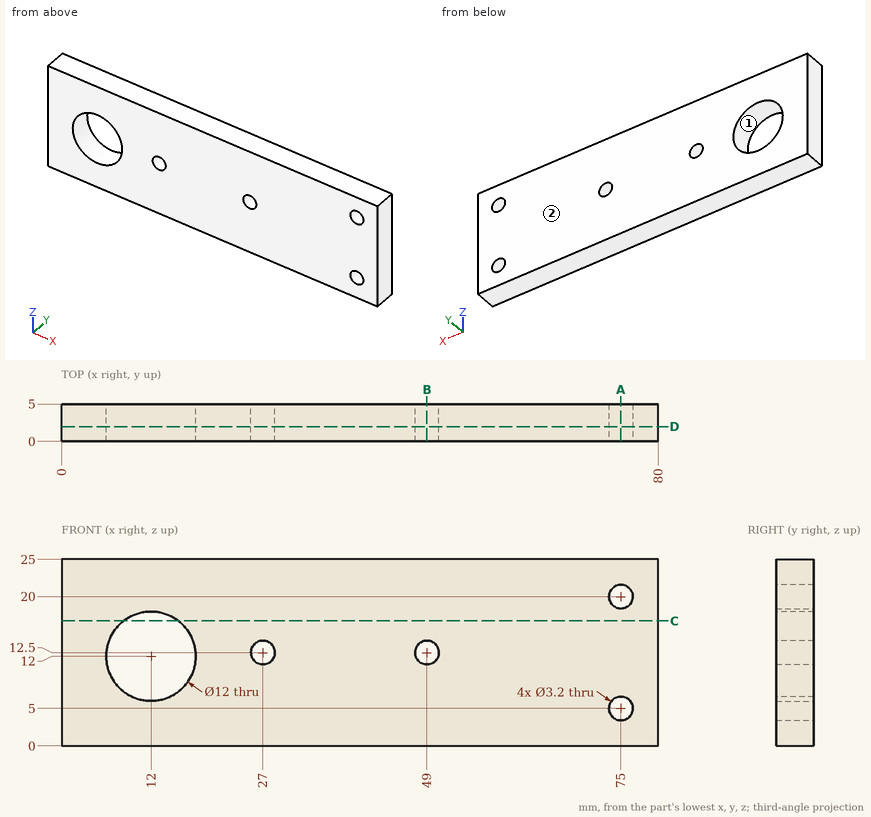
Drawing for the job (mm, zero at the part's lowest x, y, z). Coordinates: 2 decimals unless noted, no trailing zeros. Write each loop counter-clockwise with the first axis right and the second up, starting at its lowest first coordinate (ties: lowest second). Pieces come first, ordered by that corner, then holes. Notation, with made-up numbers: (-32, 69.25) - (-14, 69.25) arc R33 ccw to (-14, 98.25) - close; hole circle Ø8 at (6.25, 52.5). An arc over 180 degrees is marked (long way). Write each question's results on one line, items separated by ' | '. Start each with the question number.
1) Cut at C-C (z = 16.75). Write the cut outline in (x, y), then the cut area to 3 significant figures.
2) Cut at B-B (x = 49). Write the cut outline in (y, z).
3) Flat gauge pin, fed straight in: P1, Ø3, axis at x = 27, z = 12.5, coming from the +Y side. Where does the tip first touch, or does it go through?
4) Probe line 1 along Z through (x, y) = (75, 3.6); line 2 along X through (y, z) = (2.55, 20); line 3 along Z through (x, y) = (12, 3). List the from-to ranges inside material, lowest first. Write a range as from..to.
5) Cut at D-D (y = 1.95). Write the cut outline in (x, z).
6) Mould opens along X. For the marked faces 1 and 2 say: pulls with the +X half, pulls with the -X half, needs draft (parallel to the pull), parting line crosses it, or undercut.
7) Cut at A-A (x = 75). Write the cut outline in (y, z).
Returned:
1) outline: (0, 0) - (8.33, 0) - (8.33, 5) - (0, 5) - close; (15.67, 0) - (80, 0) - (80, 5) - (15.67, 5) - close | area: 363 mm^2
2) outline: (0, 0) - (5, 0) - (5, 10.9) - (0, 10.9) - close; (0, 14.1) - (5, 14.1) - (5, 25) - (0, 25) - close
3) P1: through
4) line 1: 0..3.4, 6.6..18.4, 21.6..25 | line 2: 0..73.4, 76.6..80 | line 3: 0..6, 18..25
5) outline: (0, 0) - (80, 0) - (80, 25) - (0, 25) - close; hole circle Ø12 at (12, 12); hole circle Ø3.2 at (27, 12.5); hole circle Ø3.2 at (49, 12.5); hole circle Ø3.2 at (75, 5); hole circle Ø3.2 at (75, 20)
6) face 1: undercut | face 2: needs draft
7) outline: (0, 0) - (5, 0) - (5, 3.4) - (0, 3.4) - close; (0, 6.6) - (5, 6.6) - (5, 18.4) - (0, 18.4) - close; (0, 21.6) - (5, 21.6) - (5, 25) - (0, 25) - close
